```python
from build123d import *

# Parameters (mm, degrees)
F1_DEPTH    = 7.5
F2_R        = 1.99999
F4_DEPTH    = 5
F5_DEPTH    = 5
F6_T1_DEPTH = 20


# Not quite as in the source:
# - a fillet or chamfer that OpenCascade refuses, or shapes differently, is made with other operations: its cross-section is extruded or revolved along the edge and cut away or added
# - a fillet or chamfer is up to 0.001 mm smaller than in the source, because OpenCascade refuses the exact size


with BuildPart() as f1:
    # F0 (on Top) → F1 (new body, symmetric)
    with BuildSketch(Plane.XY):
        Polygon((29.4704200836, 8.5355388032), (29.4704200836, 10.5355388032), (-5.5295799164, 10.5355388032), (-5.5295799164, -27.9644611968), (29.4704200836, -27.9644611968), (29.4704200836, -25.9644611968), (27.4704200836, -25.9644611968), (-3.5295799164, -25.9644611968), (-3.5295799164, 8.5355388032), (27.4704200836, 8.5355388032), align=None)
    extrude(amount=F1_DEPTH, both=True)

    # F2 (radius 2 in the source; OpenCascade refuses exactly that, so slightly less here)
    f2_edges = [f1.edges().sort_by_distance(p)[0] for p in [
        (11.97042, 10.535539, 7.5),
        (11.97042, 10.535539, -7.5),
        (-5.52958, -8.714461, 7.5),
        (29.47042, -27.964461, 0),
        (-5.52958, -27.964461, 0),
        (29.47042, 10.535539, 0),
        (-5.52958, -8.714461, -7.5),
    ]]
    fillet(f2_edges, radius=F2_R)

    # F3 (on Front) → F4 (join, symmetric)
    with BuildSketch(Plane.XZ):
        with BuildLine():
            ThreePointArc((-11.7295799164, 1.7323087668), (-9.1295799164, 4.000441756), (-6.5295799164, 1.7323087668))
            Line((-6.5295799164, 1.7323087668), (-6.5295799164, -1.7323087668))
            ThreePointArc((-6.5295799164, -1.7323087668), (-9.1295799164, -4.000441756), (-11.7295799164, -1.7323087668))
            Line((-11.7295799164, -1.7323087668), (-11.7295799164, -1.5))
            Line((-11.7295799164, -1.5), (-12.7295799164, -1.5))
            Line((-12.7295799164, -1.5), (-12.7295799164, -5.500441756))
            Line((-12.7295799164, -5.500441756), (-5.5295799164, -5.500441756))
            Line((-5.5295799164, -5.500441756), (-5.5295799164, 5.500441756))
            Line((-5.5295799164, 5.500441756), (-12.7295799164, 5.500441756))
            Line((-12.7295799164, 5.500441756), (-12.7295799164, 1.5))
            Line((-12.7295799164, 1.5), (-11.7295799164, 1.5))
            Line((-11.7295799164, 1.5), (-11.7295799164, 1.7323087668))
        make_face()
    extrude(amount=F4_DEPTH, both=True)

    # F3 (on Front) → F5 (join)
    with BuildSketch(Plane.XZ):
        with BuildLine():
            Line((-6.5295799164, -1.7323087668), (-6.5295799164, 1.7323087668))
            ThreePointArc((-6.5295799164, 1.7323087668), (-9.1295799164, 4.000441756), (-11.7295799164, 1.7323087668))
            Line((-11.7295799164, 1.7323087668), (-11.7295799164, 1.5))
            Line((-11.7295799164, 1.5), (-10.5992737621, 1.5))
            ThreePointArc((-10.5992737621, 1.5), (-8.3160558159, 1.9360213165), (-7.0295799164, 0))
            ThreePointArc((-7.0295799164, 0), (-8.3160558159, -1.9360213165), (-10.5992737621, -1.5))
            Line((-10.5992737621, -1.5), (-11.7295799164, -1.5))
            Line((-11.7295799164, -1.5), (-11.7295799164, -1.7323087668))
            ThreePointArc((-11.7295799164, -1.7323087668), (-9.1295799164, -4.000441756), (-6.5295799164, -1.7323087668))
        make_face()
    extrude(amount=F5_DEPTH)

    # F6: fillet of radius 2 on 4 edges, made by hand

    # F6_s2 → F6_t1 (cut)
    with BuildSketch(Plane.XZ.offset(-10)):
        with BuildLine():
            ThreePointArc((-12.7295799164, 3.500441756), (-12.1437934788, 4.9146553183), (-10.7295799164, 5.500441756))
            Line((-10.7295799164, 5.500441756), (-12.7295799164, 5.500441756))
            Line((-12.7295799164, 5.500441756), (-12.7295799164, 3.500441756))
        make_face()
        with BuildLine():
            ThreePointArc((-10.7295799164, -5.500441756), (-12.1437934788, -4.9146553183), (-12.7295799164, -3.500441756))
            Line((-12.7295799164, -3.500441756), (-12.7295799164, -5.500441756))
            Line((-12.7295799164, -5.500441756), (-10.7295799164, -5.500441756))
        make_face()
        with BuildLine():
            ThreePointArc((-10.7295799164, 1.5), (-12.1437934788, 2.0857864376), (-12.7295799164, 3.5))
            Line((-12.7295799164, 3.5), (-12.7295799164, 1.5))
            Line((-12.7295799164, 1.5), (-10.7295799164, 1.5))
        make_face()
        with BuildLine():
            ThreePointArc((-10.7295799164, -1.5), (-12.1437934788, -2.0857864376), (-12.7295799164, -3.5))
            Line((-12.7295799164, -3.5), (-12.7295799164, -1.5))
            Line((-12.7295799164, -1.5), (-10.7295799164, -1.5))
        make_face()
    extrude(amount=F6_T1_DEPTH, mode=Mode.SUBTRACT)


solid = f1.part
```
Can you work these out from the model? Positions are in its coordinate system, mm. A direction names the side the tool comes from. Coordinates: 2 decimals unless noted, no trailing zeros. Put each result on its own line as item: value. Start each with the question number.
(1) Will these pins go through, and if not, where does the flat tip stop? pin 1 Ø8 at (y, z) = (6, 3.5) entering from -X; pin 2 Ø5 at (y, z) = (-4, 4.5) entering from +X; pin 3 Ø8 at (x, z) = (-10.5, -2) entering from -Y; pin 4 Ø1.7 at (y, z) = (8.5, 2) entering from -X.
(2) I need wall thicknesses on probe 1 along Y at (x, z) = (24.5, 1.5); probe 2 along X at (y, z) = (-19.5, -3.25); probe 3 along Z at (x, y) = (-9, 2.5). Which ranges of each line are inside material? Lowest first, please.
(3) Which directions (+Z, -Z, +X, -X, +Y, -Y) give clear straight access to the entire face, cutting with the end or side of a thin tool? Please do faces 1 (the face through (-6.8, -5, 0.1)), 2 (the face through (-8, 0, 2)), 3 (the face through (-12.355, 0.07, 2.335)), 4 (the face through (-5.53, 8, 0)).
(4) We'd pull the mould along Z, two halves only. Please class faces 5 (the face through (-8, 0, 5.5)), 6 (the face through (13, -25.964, 0)), 7 (the face through (-12.355, 0.07, -2.335)): +Z half, -Z half, draft (parallel to the pull), parting line (faces both ways), or undercut.
Worked answers:
1. pin 1: stops at x = -12.73
1. pin 2: stops at x = -3.53
1. pin 3: stops at y = -5
1. pin 4: stops at x = -5.53
2. probe 1: y = -27.96 to -25.96, 8.54 to 10.54
2. probe 2: x = -5.53 to -3.53
2. probe 3: z = -5.5 to -4, 4 to 5.5
3. face 1: +Z, -Z, -X, -Y
3. face 2: +Y
3. face 3: -X, +Y, -Y
3. face 4: +Z, -Z, -X, +Y
4. face 5: +Z half
4. face 6: draft
4. face 7: undercut
